Check sheet for the modelled part. Datum: model origin and axes. Units: mm. Give positions to 0.01 mm unless a question says otherwise; leave off trailing zeros. Write each loop counter-clockwise with the first axis right and the second up, starting at its lowest first coordinate (ties: lowest second). Pieces come first, ordered by that corner, then holes. Notation, with made-up numbers: M 71,63 L 82,63 A29 ccw 82,97 Z; hole C 73,-5 d3. An arc over 180 degrees is marked long. Write item = value, one per line. Start each with the question number.
1) Scan lines: L1, parallel to Y at x = 0, z = 1.4; L2, parallel to Y at x = -5, z = -0.85; L3, parallel to X at y = -9, z = -0.2. Record each from-to range of solid material in increasing order.
2) Sectioned sample at A-A, the plane x = 90. Record the cut outline in (y, z), then the cut area to 3 significant figures.
3) Sectioned sample at C-C, the plane z = 0.7. Record the cut outline in (x, y), then the cut area to 3 significant figures.
4) Sectioned sample at D-D, the plane y = -90. Record the cut outline in (x, z), then the cut area to 3 significant figures.
5) Gauge pin test, flat ends, axial feed: pin 1 (2 mm diameter, centred on y = -3, z = -0.5, fed in from -X); pin 2 (3 mm diameter, centred on x = 61, z = -2, fed in from -Y); pin 3 (2.5 mm diameter, centred on x = -2.5, z = 0.5, fed in from +Y); pin 4 (5.5 mm diameter, centred on x = 0, y = -90, fed in from +Z). Record the tip position at first contact, or that the pin passes through.
6) Sectioned sample at B-B, the plane y = 0. Record the cut outline in (x, z).
from build123d import *

# Parameters (mm, degrees)
SKETCH_R  = 3.1
PAD_DEPTH = 2.5
FILLET_R  = 5


with BuildPart() as part:
    # Sketch → Pad (new body, symmetric)
    with BuildSketch(Plane.XY):
        Polygon((16, 15), (105, 15), (105, -15), (15, -105), (-15, -105), (-15, -16), (16, -16), align=None)
        with Locations((30, 0)):
            Circle(SKETCH_R, mode=Mode.SUBTRACT)
        with Locations((90, 0)):
            Circle(SKETCH_R, mode=Mode.SUBTRACT)
        with Locations((0, -30)):
            Circle(SKETCH_R, mode=Mode.SUBTRACT)
        with Locations((0, -90)):
            Circle(SKETCH_R, mode=Mode.SUBTRACT)
    extrude(amount=PAD_DEPTH, both=True)

    # Fillet
    fillet_edges = [part.edges().sort_by_distance(p)[0] for p in [
        (-15, -105, 0),
        (105, 15, 0),
        (15, -105, 0),
        (105, -15, 0),
        (16, 15, 0),
        (-15, -16, 0),
    ]]
    fillet(fillet_edges, radius=FILLET_R)


solid = part.part
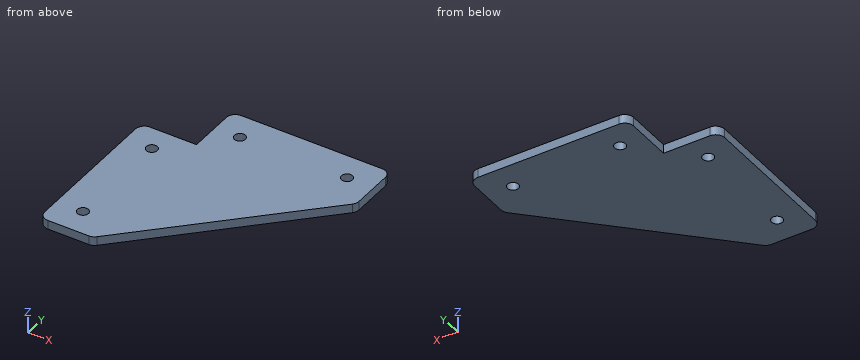
Data:
q1.L1 = -105 to -93.1, -86.9 to -33.1, -26.9 to -16
q1.L2 = -105 to -16
q1.L3 = 16 to 105
q2.outline = M -30,-2.5 L -3.1,-2.5 L -3.1,2.5 L -30,2.5 Z; M 3.1,-2.5 L 15,-2.5 L 15,2.5 L 3.1,2.5 Z
q2.area = 194 mm2
q3.outline = M -15,-100 A5 ccw -10,-105 L 12.93,-105 A5 ccw 16.46,-103.54 L 103.54,-16.46 A5 ccw 105,-12.93 L 105,10 A5 ccw 100,15 L 21,15 A5 ccw 16,10 L 16,-16 L -10,-16 A5 ccw -15,-21 Z; hole C 0,-90 d6.2; hole C 0,-30 d6.2; hole C 30,0 d6.2; hole C 90,0 d6.2
q3.area = 9,250 mm2
q4.outline = M -15,-2.5 L -3.1,-2.5 L -3.1,2.5 L -15,2.5 Z; M 3.1,-2.5 L 30,-2.5 L 30,2.5 L 3.1,2.5 Z
q4.area = 194 mm2
q5.pin_1 = 16
q5.pin_2 = -60.5
q5.pin_3 = -16
q5.pin_4 = through
q6.outline = M 16,-2.5 L 26.9,-2.5 L 26.9,2.5 L 16,2.5 Z; M 33.1,-2.5 L 86.9,-2.5 L 86.9,2.5 L 33.1,2.5 Z; M 93.1,-2.5 L 105,-2.5 L 105,2.5 L 93.1,2.5 Z
